from build123d import *

# Parameters (mm, degrees)
SKETCH_1_R      = 2
EXTRUDE_1_DEPTH = 3


with BuildPart() as part:
    # 草图1 → 凸台-拉伸1 (new body)
    with BuildSketch(Plane.XY):
        with BuildLine():
            Line((0, 2.5), (-46, 2.5))
            ThreePointArc((-46, 2.5), (-48.5, 0), (-46, -2.5))
            Line((-46, -2.5), (0, -2.5))
            ThreePointArc((0, -2.5), (2.5, 0), (0, 2.5))
        make_face()
        Circle(SKETCH_1_R, mode=Mode.SUBTRACT)
        with Locations(Location((-46, 0, 0), (0, 0, 180))):
            Circle(SKETCH_1_R, mode=Mode.SUBTRACT)
    extrude(amount=EXTRUDE_1_DEPTH)


solid = part.part
Design review of the part built by this model. Coordinates are the model's own, in mm. Give positions to 0.01 mm unless a question says otherwise; leave off trailing zeros. Loops run counter-clockwise (first coordinate to the right, second up) from the corner with the lowest first, then second, coordinate; pieces in that order, holes last. Notation, with made-up numbers: M -21.5,65.25 L -14.5,65.25 A6 cw -14.5,69.25 Z; hole C 32,46.25 d10. An arc over 180 degrees is marked long. One line per question, with ' | ' between items. Start each with the question number.
1. Add section B-B (z = 1.85). Write out the cut boundary in (x, y), plus the area to 3 significant figures.
2. The part is to be moulded in two halves that separate along X. For faces 1 (the face through (-48.5, 0.1, 1.5)), 2 (the face through (-23, 2.5, 1)), 3 (the face through (-44, 0, 1)), 4 (the face through (0, -2, 1)), say which applies: released by +X, released by -X, zero draft, split by the parting line, or undercut.
3. Add section A-A (y = 0). Write out the cut boundary in (x, z), plus the area to 3 significant figures.
4. To check wall thickness, follow L1, parallel to X at y = 0.2, z = 0.4; L2, parallel to Y at x = -46, z = 1.55; L3, parallel to X at y = -1.5, z = 1. State the ranges of each line that lie inside material, in increasing order.
5. Insertion check: P1, Ø1.5, axis at y = -1.5, z = 2.5, coming from the -X side. The pin has a flat end and moves straight along its axis. Give the tip position at first contact, or say it passes through.
Worked out:
1) outline: M -46,-2.5 L 0,-2.5 A2.5 ccw 0,2.5 L -46,2.5 A2.5 ccw Z; hole C -46,0 d4; hole C 0,0 d4 | area: 225 mm²
2) face 1: released by -X | face 2: zero draft | face 3: undercut | face 4: undercut
3) outline: M -48.5,0 L -48,0 L -48,3 L -48.5,3 Z; M -44,0 L -2,0 L -2,3 L -44,3 Z; M 2,0 L 2.5,0 L 2.5,3 L 2,3 Z | area: 129 mm²
4) L1: x = -48.49 to -47.99, -44.01 to -1.99, 1.99 to 2.49 | L2: y = -2.5 to -2, 2 to 2.5 | L3: x = -48 to -47.32, -44.68 to -1.32, 1.32 to 2
5) P1: stops at x = -48.38
